```python
from build123d import *

# Parameters (mm, degrees)
F0_W     = 60
F0_H     = 19
F1_DEPTH = 9.13
F2_R     = 9.49999
F3_W     = 13
F3_H     = 4.318
F4_DEPTH = 19.05
F5_SIZE  = 1.27
F6_R     = 5.08


# Not quite as in the source:
# - a fillet or chamfer is up to 0.001 mm smaller than in the source, because OpenCascade refuses the exact size


with BuildPart() as f1:
    # F0 (on Front) → F1 (new body, symmetric)
    with BuildSketch(Plane.XZ):
        Rectangle(F0_W, F0_H)
    extrude(amount=F1_DEPTH, both=True)

    # F2 (radius 9.5 in the source; OpenCascade refuses exactly that, so slightly less here)
    f2_edges = [f1.edges().sort_by_distance(p)[0] for p in [
        (30, 0, 9.5),
        (30, 0, -9.5),
        (-30, 0, 9.5),
        (-30, 0, -9.5),
    ]]
    fillet(f2_edges, radius=F2_R)

    # F3 (on face) → F4 (join)
    with BuildSketch(Plane(origin=(0, 9.13, 0), x_dir=(-1, 0, 0), z_dir=(0, 1, 0))):
        with Locations((-14.3949933554, 0)):
            Rectangle(F3_W, F3_H)
    extrude(amount=F4_DEPTH)

    # F5
    f5_edges = [f1.edges().sort_by_distance(p)[0] for p in [
        (14.394993, 28.18, 2.159),
        (20.894993, 28.18, 0),
        (7.894993, 28.18, 0),
        (14.394993, 28.18, -2.159),
    ]]
    chamfer(f5_edges, length=F5_SIZE)

    # F6
    f6_edges = [f1.edges().sort_by_distance(p)[0] for p in [
        (0, 9.13, 9.5),
        (0, -9.13, 9.5),
    ]]
    fillet(f6_edges, radius=F6_R)


solid = f1.part
```
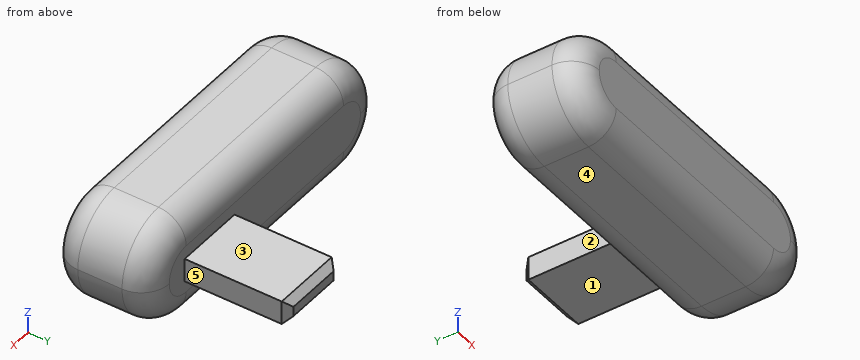
Model file for the job. Use its own axes, mm. Face numbers are marked on the shaded views. A direction names the side the tool comes from. Round coordinates to 2 decimals unless told otherwise and drop trailing zeros. Write each loop counter-clockwise with the first axis right and the second up, starting at its lowest first coordinate (ties: lowest second). Pieces come first, ordered by that corner, then holes. Notation, with made-up numbers: (72, -17.5) -> (125, -17.5) arc R25 ccw to (125, 2.5) -> close; hole circle Ø4 at (20.5, 74). An arc over 180 degrees is marked (long way). Answer as CSV lines item,"result".
1. Slice it at B-B, the plane x = -11.5. List the corners of the cut face in (y, z).
Resolved:
outline,"(-9.13, -4.42) arc R5.08 ccw to (-4.05, -9.5) -> (4.05, -9.5) arc R5.08 ccw to (9.13, -4.42) -> (9.13, 4.42) arc R5.08 ccw to (4.05, 9.5) -> (-4.05, 9.5) arc R5.08 ccw to (-9.13, 4.42) -> close"
2. Drill centre lines: line 1 (Y direction, x = 1, z = 4.75); line 2 (Z direction, x = 17.5, y = 13.5); line 3 (Y direction, x = -2, z = 7.75). Where is each one in solid material? Low to high.
Resolved:
line 1,"-9.12 to 9.12"
line 2,"-2.16 to 2.16"
line 3,"-7.89 to 7.89"
3. Slice it at D-D, the plane y = 17. List the corners of the cut face in (x, z) (3 decimals), plus the area to 3 significant figures.
Resolved:
outline,"(7.895, -2.159) -> (20.895, -2.159) -> (20.895, 2.159) -> (7.895, 2.159) -> close"
area,"56.1 mm²"
4. Pin check, flat tips, straight feed: pin 1 Ø4 at (x, y) = (13.5, -5) entering from -Z; pin 2 Ø4.5 at (y, z) = (22, -0.5) entering from +X (3 decimals); pin 3 Ø10 at (x, y) = (23, 9.5) entering from -Z; pin 4 Ø9.5 at (x, z) = (-10, 0.5) entering from +Y. Stop position of each tip, or through.
Resolved:
pin 1,"z = -9.5"
pin 2,"x = 20.895"
pin 3,"z = -9.41"
pin 4,"y = 9.13"
5. Slice it at C-C, the plane x = 16. List the corners of the cut face in (y, z).
Resolved:
outline,"(-9.13, -4.42) arc R5.08 ccw to (-4.05, -9.5) -> (4.05, -9.5) arc R5.08 ccw to (9.13, -4.42) -> (9.13, -2.16) -> (26.91, -2.16) -> (28.18, -0.89) -> (28.18, 0.89) -> (26.91, 2.16) -> (9.13, 2.16) -> (9.13, 4.42) arc R5.08 ccw to (4.05, 9.5) -> (-4.05, 9.5) arc R5.08 ccw to (-9.13, 4.42) -> close"
6. Tool access for the marked faces 1, 2, 3, 4 and 5: list every direction of +Z, -Z, +X, -X, +Y, -Y with a clear straight run to the whole face (end or side of a thin tool).
Resolved:
face 1,"-Z, +X, -X, +Y"
face 2,"+Z, -Z, -X, +Y"
face 3,"+Z, +X, -X, +Y"
face 4,"-Z, +X, -X, +Y, -Y"
face 5,"+Z, -Z, +X, +Y"
